For this review, take the finished solid that the model builds, in its own axes (mm). A direction names the side the tool comes from. Round coordinates to 2 decimals unless told otherwise and drop trailing zeros. Write each loop counter-clockwise with the first axis right and the second up, starting at its lowest first coordinate (ties: lowest second). Pieces come first, ordered by that corner, then holes.
from build123d import *

# Parameters (mm, degrees)
DOME1_FACE_RADIUS   = 8.89
DOME1_HEIGHT        = 1.27
SKETCH2_OUTSIDE_W   = 33.908
SKETCH2_OUTSIDE_H   = 33.908
CUT_EXTRUDE1_DEPTH  = 4.6736
SKETCH3_R           = 0.9525
BOSS_EXTRUDE1_DEPTH = 25.4
SKETCH4_R           = 0.635
BOSS_EXTRUDE2_DEPTH = 5.08
FILLET1_R           = 0.889
FILLET2_R           = 0.381


with BuildPart() as part:
    # Sketch1 → Revolve1 (revolve)
    with BuildSketch(Plane.XY):
        Polygon((0, 35.56), (8.89, 35.56), (8.89, 34.29), (9.9187, 33.2613), (9.9187, 28.448), (9.40435, 28.448), (9.40435, 27.94), (8.5, 27.94), (8.5, 23.9776), (11.1125, 23.9776), (11.1125, 18.669), (7.992, 18.669), (7.992, 2.286), (3.81, 2.286), (3.81, 0), (0, 0), align=None)
    revolve(axis=Axis((0, 0, 0), (0, 1, 0)))

    # Dome1: a dome of height H over a round flat face of radius A is a cap of a sphere of radius (A * A + H * H) / (2 * H)
    dome1_r = (DOME1_FACE_RADIUS * DOME1_FACE_RADIUS + DOME1_HEIGHT * DOME1_HEIGHT) / (2 * DOME1_HEIGHT)
    dome1_base = Plane((0, 35.56, 0), z_dir=(0, 1, 0))
    with Locations(dome1_base.offset(DOME1_HEIGHT - dome1_r)):
        dome1_ball = Sphere(dome1_r, mode=Mode.PRIVATE)
    add(split(dome1_ball, bisect_by=dome1_base, keep=Keep.TOP, mode=Mode.PRIVATE))

    # Sketch2 outside → Cut-Extrude1 (cut)
    with BuildSketch(Plane.XZ.offset(-18.669)):
        Rectangle(SKETCH2_OUTSIDE_W, SKETCH2_OUTSIDE_H)
        Polygon((0, 10.998522628), (-9.525, 5.499261314), (-9.525, -5.499261314), (0, -10.998522628), (9.525, -5.499261314), (9.525, 5.499261314), align=None, mode=Mode.SUBTRACT)
    extrude(amount=-CUT_EXTRUDE1_DEPTH, mode=Mode.SUBTRACT)

    # Sketch3 → Boss-Extrude1 (add)
    with BuildSketch(Plane.XZ):
        with Locations((-1.397, 0)):
            Circle(SKETCH3_R)
        with Locations((1.397, 0)):
            Circle(SKETCH3_R)
    extrude(amount=BOSS_EXTRUDE1_DEPTH)

    # Sketch4 → Boss-Extrude2 (add)
    with BuildSketch(Plane.XZ.offset(25.4)):
        with Locations((1.397, 0)):
            Circle(SKETCH4_R)
        with Locations((-1.397, 0)):
            Circle(SKETCH4_R)
    extrude(amount=BOSS_EXTRUDE2_DEPTH)

    # Fillet1
    fillet1_edges = [part.edges().sort_by_distance(p)[0] for p in [
        (-7.992, 2.286, 0),
    ]]
    fillet(fillet1_edges, radius=FILLET1_R)

    # Fillet2
    fillet2_edges = [part.edges().sort_by_distance(p)[0] for p in [
        (-3.81, 0, 0),
        (-3.81, 2.286, 0),
    ]]
    fillet(fillet2_edges, radius=FILLET2_R)


solid = part.part
(1) Mouldability with a two-part tool opening along X and no side actions: class faces 1 (the face through (4.83, 20.97, 8.21)), 2 (the face through (-2.03, -27.9, 0.03)), 3 (the face through (-4, 27.94, 8)) as pulls with the +X half, pulls with the -X half, needs draft (parallel to the pull), parting line crosses it, or undercut.
Geometry check:
face 1: pulls with the +X half
face 2: undercut
face 3: needs draft
(2) For faces 4 (the face through (-6, 23.978, 7)), 5 (the face through (-0.49, -12.52, 0.29)), 6 (the face through (-7.31, 30.821, -6.704)), list the 3-axis set-ups (+Z, -Z, +X, -X, +Y, -Y) from which the entire face can be reached by the end or side of a thin tool; tool diameter is ignored.
Geometry check:
face 4: none
face 5: -Y
face 6: +Y
(3) We need section A-A, the plane y = -21. Give the boundary of the cut face in (x, z) (1 decimal).
Geometry check:
outline: circle Ø1.9 at (-1.4, 0); circle Ø1.9 at (1.4, 0)
(4) For line 1 along Z through (x, y) = (-1.5, -20.5); line 2 along Y through (x, z) = (6.5, -5.75); line 3 along Z through (x, y) = (2, 1), list the stretches that pass through material, from the lowest coordinate up.
Geometry check:
line 1: z = -0.95 to 0.95
line 2: y = 18.67 to 23.98, 27.94 to 35.62
line 3: z = -3.24 to 3.24
(5) For pin 1 Ø3.5 at (y, z) = (20, 0.5) entering from +X (3 decimals); pin 2 Ø6 at (x, z) = (6, -7.5) entering from +Y; pin 3 Ø3 at (x, y) = (-7.5, 28) entering from +Z, all flat-tipped, find the tip position at first contact; note any pin that passes through.
Geometry check:
pin 1: stops at x = 9.525
pin 2: stops at y = 36.14
pin 3: stops at z = 7.85
(6) We need section C-C, the plane y = 5.5. Give the boundary of the cut face in (x, z), and give its area (3 significant figures).
Geometry check:
outline: circle Ø15.98 at (0, 0)
area: 201 mm2
(7) We need section B-B, the plane y = 25.5. Give the boundary of the cut face in (x, z).
Geometry check:
outline: circle Ø17 at (0, 0)
